The listing builds one solid part. Answer for the finished solid, in the listing's coordinates (mm). Coordinates: 2 decimals unless noted, no trailing zeros. Loops run counter-clockwise (first coordinate to the right, second up) from the corner with the lowest first, then second, coordinate; pieces in that order, holes last. Notation, with made-up numbers: (4, 45) -> (32, 45) arc R21 cw to (32, 80) -> close; hole circle Ø1 at (41.5, -32.5). An arc over 180 degrees is marked (long way). Answer in a Markdown table with one row per item.
```python
from build123d import *

# Parameters (mm, degrees)
SKETCH1_R           = 28
SKETCH1_R_2         = 20
BOSS_EXTRUDE1_DEPTH = 0.254
CIRPATTERN1_COUNT   = 8


with BuildPart() as part:
    # Sketch1 → Boss-Extrude1 (new body)
    with BuildSketch(Plane.XY):
        Circle(SKETCH1_R)
        Circle(SKETCH1_R_2, mode=Mode.SUBTRACT)
    extrude(amount=BOSS_EXTRUDE1_DEPTH)

    # Sketch2 → 2.5 _2.5_ Diameter Hole1 (revolve, cut)
    with BuildSketch(Plane(origin=(0, 24, 0.254), x_dir=(0, -1, 0), z_dir=(1, 0, 0))):
        Polygon((0, 0), (0, 2.251075774), (1.25, 1.5), (1.25, 0), align=None)
    f_2_5_2_5_diameter_hole1 = revolve(axis=Axis((0, 24, 6.604), (0, 0, -1)), mode=Mode.SUBTRACT)

    # CirPattern1: 2.5 _2.5_ Diameter Hole1 ×8 about axis
    cirpattern1_axis = Axis((0, 0, 0), (0, 0, 1))
    for i in range(1, CIRPATTERN1_COUNT):
        add(f_2_5_2_5_diameter_hole1.rotate(cirpattern1_axis, i * 360 / CIRPATTERN1_COUNT), mode=Mode.SUBTRACT)


solid = part.part
```
Item 1: A cutting plane is placed at D-D, the plane z = 0.2. Count the separate pieces of the cut face and the enclosed holes in it, plus the area to 3 significant figures.
Findings below:
| item | result |
|---|---|
| separate pieces | 1 |
| enclosed holes | 9 |
| area | 1,170 mm2 |
Item 2: A cutting plane is placed at A-A, the plane x = 0. Determine the outline of the cut face in (y, z).
Findings below:
| item | result |
|---|---|
| outline | (-28, 0) -> (-25.25, 0) -> (-25.25, 0.25) -> (-28, 0.25) -> close; (-22.75, 0) -> (-20, 0) -> (-20, 0.25) -> (-22.75, 0.25) -> close; (20, 0) -> (22.75, 0) -> (22.75, 0.25) -> (20, 0.25) -> close; (25.25, 0) -> (28, 0) -> (28, 0.25) -> (25.25, 0.25) -> close |
Item 3: Find the intervals of material crossed by probe 1 along Y at (x, z) = (0, 0.2); probe 2 along X at (y, z) = (-16, 0.1); probe 3 along Y at (x, z) = (-9, 0.2), in increasing order.
Findings below:
| item | result |
|---|---|
| probe 1 | y = -28 to -25.25, -22.75 to -20, 20 to 22.75, 25.25 to 28 |
| probe 2 | x = -22.98 to -17.76, -16.18 to -12, 12 to 16.18, 17.76 to 22.98 |
| probe 3 | y = -26.51 to -17.86, 17.86 to 26.51 |
Item 4: A cutting plane is placed at C-C, the plane x = 10.5. Determine the outline of the cut face in (y, z).
Findings below:
| item | result |
|---|---|
| outline | (-25.96, 0) -> (-17.02, 0) -> (-17.02, 0.25) -> (-25.96, 0.25) -> close; (17.02, 0) -> (25.96, 0) -> (25.96, 0.25) -> (17.02, 0.25) -> close |
